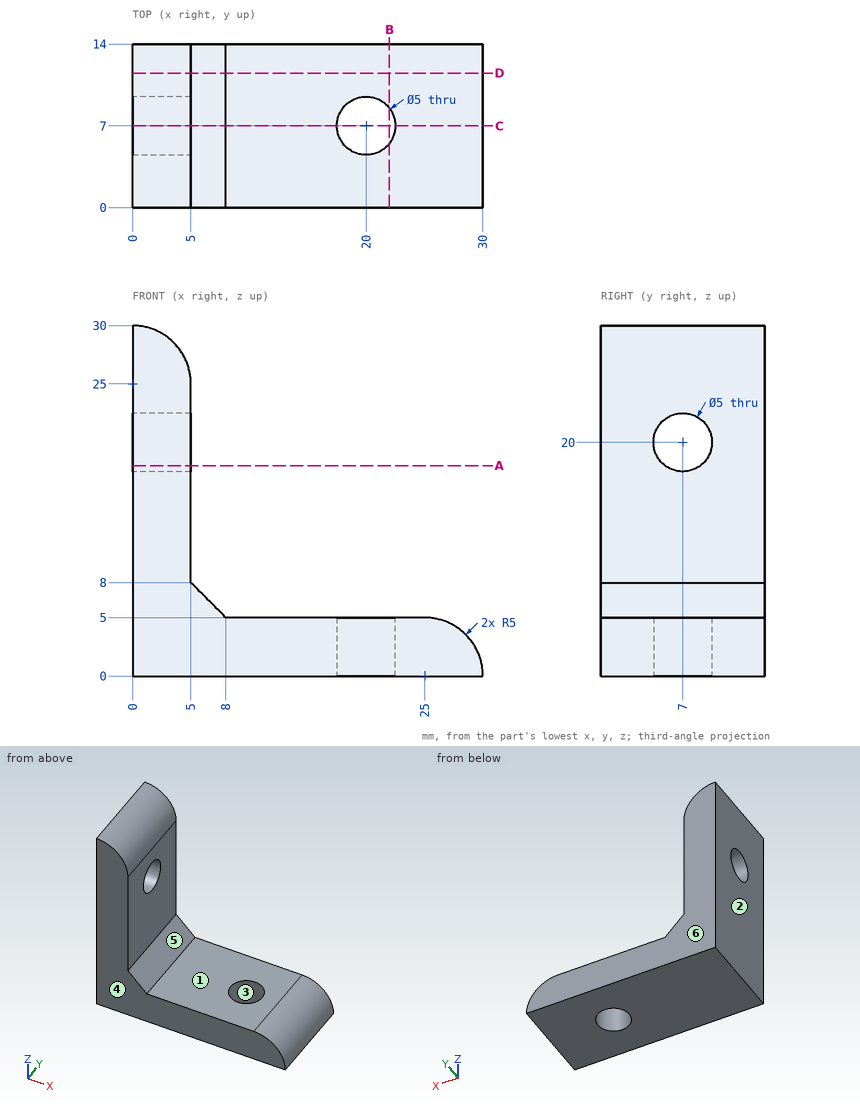
Source: three-view drawing plus pictorial views. Frame: mm from the lowest corner of the part. A direction names the side the tool comes from. Give positions to 0.01 mm unless a question says otherwise; leave off trailing zeros. Loops run counter-clockwise (first coordinate to the right, second up) from the corner with the lowest first, then second, coordinate; pieces in that order, holes last.
1) Section query D-D on y = 11.5. Return the cut outline in (x, z).
A:
outline: (0, 0) - (30, 0) arc R5 ccw to (25, 5) - (8, 5) - (5, 8) - (5, 25) arc R5 ccw to (0, 30) - close
2) Line query: L1, parallel to Y at x = 20, z = 1.6; L2, parallel to Z at x = 25, y = 3.75; L3, parallel to Z at x = 1.7, y = 7. Output: solid intervals per line, ascending.
A:
L1: y = 0 to 4.5, 9.5 to 14
L2: z = 0 to 5
L3: z = 0 to 17.5, 22.5 to 29.7
3) Section query C-C on y = 7. Return the cut outline in (x, z).
A:
outline: (0, 0) - (17.5, 0) - (17.5, 5) - (8, 5) - (5, 8) - (5, 17.5) - (0, 17.5) - close; (0, 22.5) - (5, 22.5) - (5, 25) arc R5 ccw to (0, 30) - close; (22.5, 0) - (30, 0) arc R5 ccw to (25, 5) - (22.5, 5) - close
4) Section query B-B on x = 22. Return the cut outline in (y, z), and give its area (3 significant figures).
A:
outline: (0, 0) - (5.5, 0) - (5.5, 5) - (0, 5) - close; (8.5, 0) - (14, 0) - (14, 5) - (8.5, 5) - close
area: 55.0 mm2
5) Contact query for flat-ended pins moving along their axis: pin 1 (3 mm diameter, centred on y = 11, z = 25, fed in from +X); pin 2 (5 mm diameter, centred on x = 23.5, y = 7, fed in from +Z); pin 3 (4 mm diameter, centred on y = 3, z = 7.5, fed in from +X). Output: stop coordinate, or through.
A:
pin 1: stops at x = 5
pin 2: stops at z = 5
pin 3: stops at x = 7.5
6) Reachability of the marked faces 1 and 2 from +Z, -Z, +X, -X, +Y, -Y: full face, straight path, thin tool, end or side. Return the list, or none.
A:
face 1: +Z, +X, +Y, -Y
face 2: +Z, -Z, -X, +Y, -Y
7) Mould query, pull axis Y, two halves, no side actions, for the marked faces 3, 4, 5 and 6. Classes: released by +Y, released by -Y, zero draft, split by the parting line, or undercut.
A:
face 3: undercut
face 4: released by -Y
face 5: zero draft
face 6: released by +Y
8) Section query A-A on z = 18. Return the cut outline in (x, y).
A:
outline: (0, 0) - (5, 0) - (5, 5.5) - (0, 5.5) - close; (0, 8.5) - (5, 8.5) - (5, 14) - (0, 14) - close
